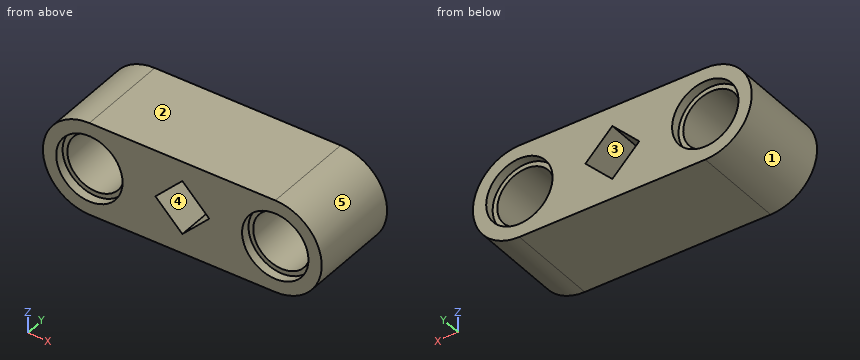
Autodesk Inventor part; units mm, degrees
ref_plane "YZ Plane" through (0, 0, 0) normal (1, 0, 0) x (0, 1, 0)
ref_plane "XZ Plane" through (0, 0, 0) normal (0, 1, 0) x (-1, 0, 0)
ref_plane "XY Plane" through (0, 0, 0) normal (0, 0, 1) x (1, 0, 0)
sketch "Sketch1" plane through (0, 0, 0) normal (0, 1, 0) x (-1, 0, 0)
  line L0 (-8.001, 0) -> (8.001, 0) construction
  line L1 (-8.001, -4.0005) -> (8.001, -4.0005)
  line L2 (8.001, 4.0005) -> (-8.001, 4.0005)
  arc A0 (-8.001, 4.0005) -> (-8.001, -4.0005) centre (-8.001, 0) ccw
  arc A1 (8.001, -4.0005) -> (8.001, 4.0005) centre (8.001, 0) ccw
  line L3 (-2.3169, 0) -> (0, 2.3169)
  line L4 (0, 2.3169) -> (2.3169, 0)
  line L5 (2.3169, 0) -> (0, -2.3169)
  line L6 (0, -2.3169) -> (-2.3169, 0)
  line L7 (-2.3169, 0) -> (2.3169, 0) construction
  line L8 (0, 2.3169) -> (0, -2.3169) construction
  point P0 (0, 0)
  dimension "d0" = 8.001
  dimension "d1" = 8.001
  dimension "d2" = 3.2766
  dimension "d3" = 3.2766
extrude "Extrusion1" add sketch "Sketch1" along normal blind 8.001
sketch "Sketch2" plane through (0, 8.001, 0) normal (0, 1, 0) x (1, 0, 0)
  circle A0 centre (-8.001, 0) radius 2.8575
  point P0 (0, 0)
  dimension "d6" = 8.001
  dimension "d7" = 5.715
extrude "Extrusion2" cut sketch "Sketch2" against normal blind 0.7874
sketch "Sketch3" plane through (0, 8.001, 0) normal (0, 1, 0) x (1, 0, 0)
  circle A0 centre (8.001, 0) radius 2.8575
  point P0 (0, 0)
  dimension "d10" = 8.001
  dimension "d11" = 5.715
extrude "Extrusion3" cut sketch "Sketch3" against normal blind 0.7874
sketch "Sketch4" plane through (0, 0, 0) normal (0, -1, 0) x (1, 0, 0)
  circle A0 centre (8.001, 0) radius 2.8575
  circle A1 centre (8.001, 0) radius 2.8575
  point P0 (0, 0)
extrude "Extrusion4" cut sketch "Sketch4" against normal blind 0.7874
sketch "Sketch5" plane through (0, 0, 0) normal (0, -1, 0) x (1, 0, 0)
  circle A0 centre (-8.001, 0) radius 2.8575
  circle A1 centre (-8.001, 0) radius 2.8575
  point P0 (0, 0)
extrude "Extrusion5" cut sketch "Sketch5" against normal blind 0.7874
sketch "Sketch6" plane through (-8.001, 7.2136, 0) normal (0, 1, 0) x (1, 0, 0)
  circle A0 centre (0, 0) radius 2.4511
  point P0 (8.001, 0)
  dimension "d18" = 4.9022
extrude "Extrusion6" cut sketch "Sketch6" against normal through all
sketch "Sketch7" plane through (8.001, 7.2136, 0) normal (0, 1, 0) x (1, 0, 0)
  circle A0 centre (0, 0) radius 2.4511
  point P0 (-8.001, 0)
  dimension "d21" = 4.9022
extrude "Extrusion7" cut sketch "Sketch7" against normal through all
properties part number "VexLegoCouplerBasic"
Read the model definition and answer for the solid it produces. Units are mm, in the model's axes. Face numbers are marked on the shaded views. A direction names the side the tool comes from. Round coordinates to 2 decimals unless told otherwise and drop trailing zeros. Order: outer loops, then holes, each group sorted by start corner. A loop starts at its lowest first (then second) coordinate and runs counter-clockwise, first axis right, second up.
1) Straight lines are drawn through the part: L1, parallel to X at y = 7, z = -1.25; L2, parallel to X at y = 2.75, z = 1.75; L3, parallel to Z at x = 9.5, y = 6.5. For each, find the intervals that lie inside material, in ascending order.
2) The part is cut by section A-A on y = 4.5. Write down the section's boundary in (x, z).
3) The part is cut by section B-B on x = -8.25. Write down the section's boundary in (y, z), plus the area to 3 significant figures.
4) The part is cut by section C-C on z = 1. Give the number of separate pieces and of enclosed holes in the cut face, plus the area to 3 significant figures.
5) The mould has two halves that part along Z. Classify the marked faces 1, 2 and 3: released by +Z, released by -Z, zero draft, split by the parting line, or undercut.
6) The part is cut by section D-D on x = 10. Write down the section's boundary in (y, z).
7) For the marked faces 4 and 5, determine the directions among +Z, -Z, +X, -X, +Y, -Y from which every point of the face is accessible in a straight line to the end or side of a thin tool.
Resolved:
1. L1: x = -11.8 to -10.11, -5.89 to -1.07, 1.07 to 5.89, 10.11 to 11.8
1. L2: x = -11.6 to -9.72, -6.28 to -0.57, 0.57 to 6.28, 9.72 to 11.6
1. L3: z = -3.71 to -1.94, 1.94 to 3.71
2. outline: (-8, -4) - (8, -4) arc R4 ccw to (8, 4) - (-8, 4) arc R4 ccw to start; hole circle Ø4.9 at (-8, 0); hole (-2.32, 0) - (0, -2.32) - (2.32, 0) - (0, 2.32) - close; hole circle Ø4.9 at (8, 0)
3. outline: (0, -3.99) - (8, -3.99) - (8, -2.85) - (7.21, -2.85) - (7.21, -2.44) - (0.79, -2.44) - (0.79, -2.85) - (0, -2.85) - close; (0, 2.85) - (0.79, 2.85) - (0.79, 2.44) - (7.21, 2.44) - (7.21, 2.85) - (8, 2.85) - (8, 3.99) - (0, 3.99) - close
3. area: 23.6 mm2
4. separate pieces: 4
4. enclosed holes: 0
4. area: 94.6 mm2
5. face 1: split by the parting line
5. face 2: released by +Z
5. face 3: undercut
6. outline: (0, -3.47) - (8, -3.47) - (8, -2.04) - (7.21, -2.04) - (7.21, -1.42) - (0.79, -1.42) - (0.79, -2.04) - (0, -2.04) - close; (0, 2.04) - (0.79, 2.04) - (0.79, 1.42) - (7.21, 1.42) - (7.21, 2.04) - (8, 2.04) - (8, 3.47) - (0, 3.47) - close
7. face 4: +Y, -Y
7. face 5: +X, +Y, -Y
